```python
from build123d import *

# Parameters (mm, degrees)
F0_W     = 450
F0_H     = 650
F1_DEPTH = 600
F2_W     = 100
F2_H     = 70
F6_R     = 20


with BuildPart() as f1:
    # F0 (on Top) → F1 (new body)
    with BuildSketch(Plane.XY):
        with Locations((225, 325)):
            Rectangle(F0_W, F0_H)
    extrude(amount=F1_DEPTH)

    # F5: sweep along a path in F4
    with BuildLine(Plane.YZ.offset(225)) as f5_path:
        Line((650, 600), (478.9899283372, 1069.846310393))
        Line((478.9899283372, 1069.846310393), (328.9899283372, 1069.846310393))
    # F2 (on face) → F5 (sweep)
    with BuildSketch(Plane.XY.offset(600)):
        with Locations((225, 615)):
            Rectangle(F2_W, F2_H)
    sweep(path=f5_path.line, transition=Transition.RIGHT)

    # F6
    f6_edges = [f1.edges().sort_by_distance(p)[0] for p in [
        (225, 478.989928, 1069.84631),
        (225, 432.931338, 1004.067827),
    ]]
    fillet(f6_edges, radius=F6_R)


solid = f1.part
```
Design review of the part built by this model. Coordinates are the model's own, in mm. A direction names the side the tool comes from. Give positions to 0.01 mm unless a question says otherwise; leave off trailing zeros. Order: outer loops, then holes, each group sorted by start corner. A loop starts at its lowest first (then second) coordinate and runs counter-clockwise, first axis right, second up. Notation, with made-up numbers: (61.25, 3) -> (86.25, 3) arc R30 ccw to (86.25, 33) -> close; hole circle Ø9 at (45, 16.25). An arc over 180 degrees is marked (long way). Write each question's results on one line, items separated by ' | '. Start each with the question number.
Q1. Machinability: for faces 4 (the flat face through (175, 491, 871)), 5 (the flat face through (450, 320, 296)), 6 (the flat face through (224.3, 507.865, 798.19)), 7 (the flat face through (226, 396, 1069.846)), 8 (the flat face through (275, 502, 871)), which of the approach directions +Z, -Z, +X, -X, +Y, -Y give a long, thin tool a straight path to every point of the face, cutting with its end or side? Answer none if there is none.
Q2. Add section B-B on x = 363. Give the boundary of the cut face in (y, z).
Q3. Wall thickness on L1, parallel to Z at x = 133.5, y = 595.5; L2, parallel to Y at x = 236.5, z = 972: over which ranges is each line inside the solid? List them lowest first. Write a range as from..to.
Q4. Mouldability with a two-part tool opening along Z and no side actions: class faces 1 (the flat face through (222, 650, 296)), 2 (the flat face through (224, 361, 1004.068)), 3 (the flat face through (225.7, 565.726, 831.54)) as +Z half, -Z half, draft (parallel to the pull), parting line (faces both ways), or undercut.
Q5. Add section A-A on y = 178. Give the boundary of the cut face in (x, z), and give its area (3 significant figures).
Q6. For pin 1 (5 mm diameter, centred on x = 106.5, y = 443, fed in from +Z), flat-tipped, find the tip position at first contact; note if it passes through.
Found:
1) face 4: +Z, -X, +Y, -Y | face 5: +Z, -Z, +X, +Y, -Y | face 6: +X, -X, -Y | face 7: +Z, +X, -X, +Y, -Y | face 8: +Z, +X, +Y, -Y
2) outline: (0, 0) -> (650, 0) -> (650, 600) -> (0, 600) -> close
3) L1: z = 0..600 | L2: y = 444.6..514.6
4) face 1: draft | face 2: undercut | face 3: +Z half
5) outline: (0, 0) -> (450, 0) -> (450, 600) -> (0, 600) -> close | area: 270,000 mm2
6) pin 1: stops at z = 600
